The drawing under review shows one solid part. Ordinate dimensions are in mm from its lowest x, y, z. Round coordinates to 2 decimals unless told otherwise and drop trailing zeros. Write each loop counter-clockwise with the first axis right and the second up, starting at its lowest first coordinate (ties: lowest second). Pieces come first, ordered by that corner, then holes. Notation, with made-up numbers: (18, 54.5) -> (68, 54.5) arc R23 cw to (68, 63.5) -> close; hole circle Ø9 at (36.25, 73). An arc over 180 degrees is marked (long way). Use CSV: the item, a comma, the result in double quotes. Start each with the question number.
1) Take a section at A-A, the plane y = 0.7. Give the boundary of the cut face in (x, z).
2) For pin 1 Ø3.5 at (x, z) = (46.5, 20) entering from +Y, flat-tipped, find the tip position at first contact; note if it passes through.
3) Take a section at B-B, the plane x = 41.75. Give the boundary of the cut face in (y, z), then the cut area to 3 significant figures.
4) Take a section at C-C, the plane z = 20. Give the boundary of the cut face in (x, y).
5) Wall thickness on probe 1 along X at (y, z) = (1.45, 20); probe 2 along X at (y, z) = (2, 5); probe 3 along Z at (x, y) = (41.75, 0.7): over which ranges is each line inside the solid? List them lowest first. Write a range as [from, to].
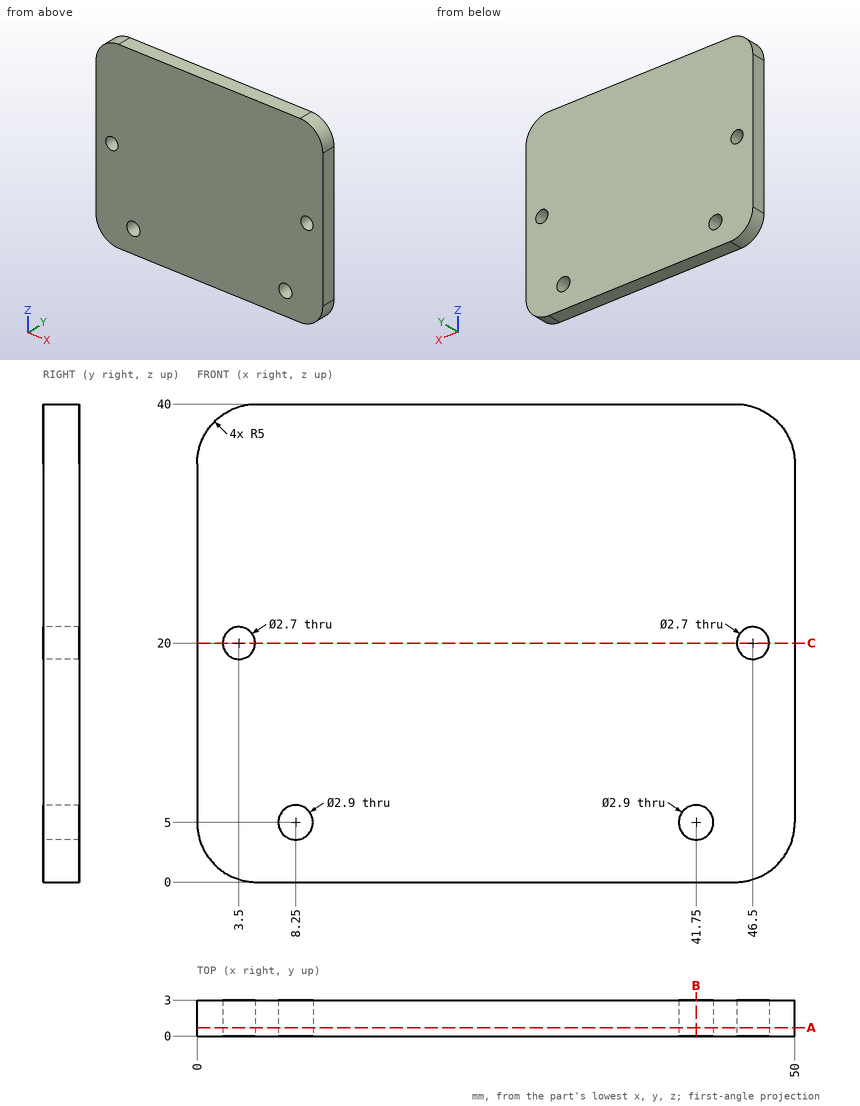
Values found:
1,outline,"(0, 5) arc R5 ccw to (5, 0) -> (45, 0) arc R5 ccw to (50, 5) -> (50, 35) arc R5 ccw to (45, 40) -> (5, 40) arc R5 ccw to (0, 35) -> close; hole circle Ø2.7 at (3.5, 20); hole circle Ø2.9 at (8.25, 5); hole circle Ø2.9 at (41.75, 5); hole circle Ø2.7 at (46.5, 20)"
2,pin 1,"y = 3"
3,outline,"(0, 0) -> (3, 0) -> (3, 3.55) -> (0, 3.55) -> close; (0, 6.45) -> (3, 6.45) -> (3, 40) -> (0, 40) -> close"
3,area,"111 mm²"
4,outline,"(0, 0) -> (2.15, 0) -> (2.15, 3) -> (0, 3) -> close; (4.85, 0) -> (45.15, 0) -> (45.15, 3) -> (4.85, 3) -> close; (47.85, 0) -> (50, 0) -> (50, 3) -> (47.85, 3) -> close"
5,probe 1,"[0, 2.15], [4.85, 45.15], [47.85, 50]"
5,probe 2,"[0, 6.8], [9.7, 40.3], [43.2, 50]"
5,probe 3,"[0, 3.55], [6.45, 40]"
